Geometry check sheet. Reference: the model listing, model coordinates, mm. Face numbers are marked on the shaded views. A direction names the side the tool comes from. Coordinates: 2 decimals unless noted, no trailing zeros. Order: outer loops, then holes, each group sorted by start corner. A loop starts at its lowest first (then second) coordinate and runs counter-clockwise, first axis right, second up. Notation, with made-up numbers: (-17.75, -13) - (-1.75, -13) arc R25 cw to (-1.75, 18) - close; hole circle Ø7 at (72, 50.25). An arc over 180 degrees is marked (long way). Put each result on its own line as item: value.
from build123d import *

# Parameters (mm, degrees)
PAD_DEPTH    = 10
SKETCH001_R  = 10
PAD001_DEPTH = 40


with BuildPart() as part:
    # Sketch → Pad (new body)
    with BuildSketch(Plane.XY):
        with BuildLine():
            ThreePointArc((13.228757, -15), (20, 0), (13.228757, 15))
            Line((-13.228757, 15), (13.228757, 15))
            ThreePointArc((-13.228757, 15), (-20, 0), (-13.228757, -15))
            Line((-13.228757, -15), (13.228757, -15))
        make_face()
    extrude(amount=PAD_DEPTH)

    # Sketch001 → Pad001 (join)
    with BuildSketch(Plane.XY):
        Circle(SKETCH001_R)
    extrude(amount=-PAD001_DEPTH)


solid = part.part
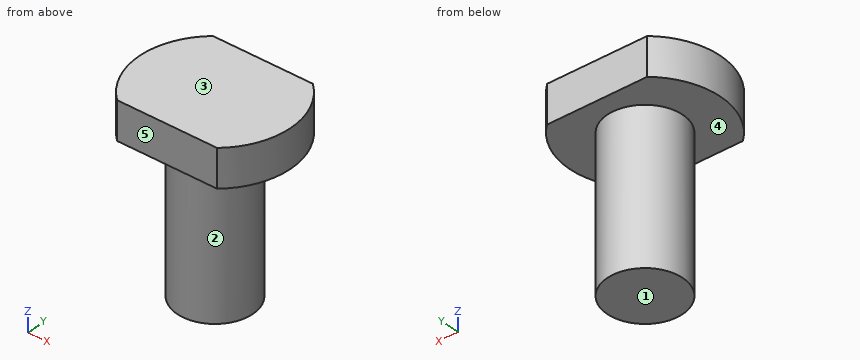
Q1. Draft check along Z on the marked faces 3, 4 and 5. Enter one of: pulls with the +Z half, pulls with the -Z half, needs draft (parallel to the pull), parting line crosses it, or undercut.
Answer block:
face 3: pulls with the +Z half
face 4: pulls with the -Z half
face 5: needs draft
Q2. Section check A-A on y = -9. Record the boundary of the cut face in (x, z).
Answer block:
outline: (-17.86, 0) - (-4.36, 0) - (-4.36, -40) - (4.36, -40) - (4.36, 0) - (17.86, 0) - (17.86, 10) - (-17.86, 10) - close
Q3. Section check D-D on y = -12. Record the boundary of the cut face in (x, z), then the cut area to 3 significant figures.
Answer block:
outline: (-16, 0) - (16, 0) - (16, 10) - (-16, 10) - close
area: 320 mm^2
Q4. Section check B-B on x = 0. Record the boundary of the cut face in (y, z), then the cut area to 3 significant figures.
Answer block:
outline: (-15, 0) - (-10, 0) - (-10, -40) - (10, -40) - (10, 0) - (15, 0) - (15, 10) - (-15, 10) - close
area: 1,100 mm^2
Q5. Section check C-C on z = -8.5. Record the boundary of the cut face in (x, y).
Answer block:
outline: circle Ø20 at (0, 0)
Q6. Thickness scan on L1, parallel to Z at x = 1, y = 12; L2, parallel to X at y = -4, z = -34.5; L3, parallel to Y at x = -0.5, z = -35. Record the ranges inside material, lowest first. Write a range as [from, to].
Answer block:
L1: z = [0, 10]
L2: x = [-9.17, 9.17]
L3: y = [-9.99, 9.99]
Q7. Access from +Z, -Z, +X, -X, +Y, -Y to the whole of each face (thin tool, end or side, straight path). Record for the marked faces 1 and 2.
Answer block:
face 1: -Z, +X, -X, +Y, -Y
face 2: -Z
Q8. Depth check by flat-ended pin: pin 1 Ø12 at (y, z) = (3.5, -24.5) entering from +X; pin 2 Ø8 at (y, z) = (-4.5, 1) entering from +X; pin 3 Ø3 at (x, z) = (3.5, -32) entering from +Y; pin 4 Ø1 at (y, z) = (-12, -31.5) entering from -X. Enter the tip coordinate at first touch or a pass-through.
Answer block:
pin 1: stops at x = 10
pin 2: stops at x = 19.99
pin 3: stops at y = 9.8
pin 4: passes through
